Design review of the part built by this model. Coordinates are the model's own, in mm. A direction names the side the tool comes from. Coordinates: 2 decimals unless noted, no trailing zeros. Loops run counter-clockwise (first coordinate to the right, second up) from the corner with the lowest first, then second, coordinate; pieces in that order, holes last.
Q1. Add section A-A on x = -4. Give the boundary of the cut face in (y, z).
Q2. For P1, Ø0.8, axis at x = 57.5, y = -25.5, coming from the -Z side, flat-tipped, find the tip position at first contact; note if it passes through.
Q3. Wall thickness on probe 1 along X at (y, z) = (28, 16.25); probe 2 along Y at (x, z) = (-52, 13.5); probe 3 along Z at (x, y) = (27, -41.5): over which ranges is each line inside the solid? List them lowest first.
Q4. Add section B-B on z = 20.25. Give the boundary of the cut face in (x, y).
Q5. Add section D-D on y = -36. Give the boundary of the cut face in (x, z), and give its area (3 significant figures).
Q6. Draft analysis for pull direction Y (two halves, no side actions). For faces 4 (the face through (-57, -42.7, 15)), 5 (the face through (-57, -8, 17.8)), 6 (the face through (-54, 32, 12.8)), 7 (the face through (0, -50.5, 19)), state which applies: released by +Y, released by -Y, zero draft, split by the parting line, or undercut.
Q7. Machinability: for faces 1 (the face through (1, 34.5, 19)), 2 (the face through (0, -47.7, 19)), 3 (the face through (-57, 26.7, 15)), which of the approach directions +Z, -Z, +X, -X, +Y, -Y give a long, thin tool a straight path to every point of the face, cutting with its end or side? Answer none if there is none.
Q8. Add section C-C on y = -16. Give the boundary of the cut face in (x, z).
```python
from build123d import *

# Parameters (mm, degrees)
SKETCH022_W     = 117
SKETCH022_H     = 85
PAD013_DEPTH    = 5.8
SKETCH023_W     = 95.2
SKETCH023_H     = 58.2
POCKET001_DEPTH = 5.801
SKETCH024_W     = 111.4
SKETCH024_H     = 79.4
POCKET002_DEPTH = 3.8
POCKET008_DEPTH = 5.801
PAD017_DEPTH    = 5
SKETCH044_W     = 2.8
SKETCH044_H     = 3.2
PAD018_DEPTH    = 1.4
SKETCH045_W     = 2.8
SKETCH045_H     = 3.2
PAD019_DEPTH    = 1.4
POCKET016_DEPTH = 85.001
CHAMFER001_SIZE = 1.4


with BuildPart() as part:
    # Sketch022 → Pad013 (new body)
    with BuildSketch(Plane.XY.offset(23.6)):
        with Locations((0.5, -8)):
            Rectangle(SKETCH022_W, SKETCH022_H)
    extrude(amount=-PAD013_DEPTH)

    # Sketch023 (on Face5 of Pad013) → Pocket001 (cut, through all)
    with BuildSketch(Plane.XY.offset(23.6)):
        with Locations((0.9, 0)):
            Rectangle(SKETCH023_W, SKETCH023_H)
    extrude(amount=-POCKET001_DEPTH, mode=Mode.SUBTRACT)

    # Sketch024 (on Face5 of Pocket001) → Pocket002 (cut)
    with BuildSketch(Plane(origin=(0, 0, 17.8), x_dir=(1, 0, 0), z_dir=(0, 0, -1))):
        with Locations((0.5, 8)):
            Rectangle(SKETCH024_W, SKETCH024_H)
    extrude(amount=-POCKET002_DEPTH, mode=Mode.SUBTRACT)

    # Sketch031 (on Face4 of Pocket002) → Pocket008 (cut, through all)
    with BuildSketch(Plane.XY.offset(23.6)):
        with BuildLine():
            Line((-51.4, -33.8), (-41.6, -33.8))
            ThreePointArc((-40.6, -34.8), (-40.892893, -34.092893), (-41.6, -33.8))
            Line((-40.6, -34.8), (-40.6, -44.6))
            ThreePointArc((-41.6, -45.6), (-40.892893, -45.307107), (-40.6, -44.6))
            Line((-41.6, -45.6), (-51.4, -45.6))
            ThreePointArc((-52.4, -44.6), (-52.107107, -45.307107), (-51.4, -45.6))
            Line((-52.4, -44.6), (-52.4, -34.8))
            ThreePointArc((-51.4, -33.8), (-52.107107, -34.092893), (-52.4, -34.8))
        make_face()
        with BuildLine():
            Line((-37.6, -33.8), (-27.8, -33.8))
            ThreePointArc((-26.8, -34.8), (-27.092893, -34.092893), (-27.8, -33.8))
            Line((-26.8, -34.8), (-26.8, -44.6))
            ThreePointArc((-27.8, -45.6), (-27.092893, -45.307107), (-26.8, -44.6))
            Line((-27.8, -45.6), (-37.6, -45.6))
            ThreePointArc((-38.6, -44.6), (-38.307107, -45.307107), (-37.6, -45.6))
            Line((-38.6, -44.6), (-38.6, -34.8))
            ThreePointArc((-37.6, -33.8), (-38.307107, -34.092893), (-38.6, -34.8))
        make_face()
        with BuildLine():
            Line((-9.5, -33.8), (0.3, -33.8))
            ThreePointArc((1.3, -34.8), (1.007107, -34.092893), (0.3, -33.8))
            Line((1.3, -34.8), (1.3, -44.6))
            ThreePointArc((0.3, -45.6), (1.007107, -45.307107), (1.3, -44.6))
            Line((0.3, -45.6), (-9.5, -45.6))
            ThreePointArc((-10.5, -44.6), (-10.207107, -45.307107), (-9.5, -45.6))
            Line((-10.5, -44.6), (-10.5, -34.8))
            ThreePointArc((-9.5, -33.8), (-10.207107, -34.092893), (-10.5, -34.8))
        make_face()
    extrude(amount=-POCKET008_DEPTH, mode=Mode.SUBTRACT)

    # Sketch038 (on Face5 of Pocket008) → Pad017 (join)
    with BuildSketch(Plane(origin=(0, 0, 17.8), x_dir=(1, 0, 0), z_dir=(0, 0, -1))):
        Polygon((-58, 50.5), (-48.2, 50.5), (-48.2, 47.7), (-55.2, 47.7), (-55.2, 42.7), (-58, 42.7), align=None)
        Polygon((59, 50.5), (49.2, 50.5), (49.2, 47.7), (56.2, 47.7), (56.2, 42.7), (59, 42.7), align=None)
        Polygon((59, -34.5), (49.2, -34.5), (49.2, -31.7), (56.2, -31.7), (56.2, -26.7), (59, -26.7), align=None)
        Polygon((-58, -34.5), (-48.2, -34.5), (-48.2, -31.7), (-55.2, -31.7), (-55.2, -26.7), (-58, -26.7), align=None)
    extrude(amount=PAD017_DEPTH)

    # Sketch044 (on Face66 of Pad017) → Pad018 (join)
    with BuildSketch(Plane.YZ.offset(-48.2)):
        with Locations((-49.1, 14.4)):
            Rectangle(SKETCH044_W, SKETCH044_H)
        with Locations((33.1, 14.4)):
            Rectangle(SKETCH044_W, SKETCH044_H)
    extrude(amount=PAD018_DEPTH)

    # Sketch045 (on Face68 of Pad018) → Pad019 (join)
    with BuildSketch(Plane(origin=(49.2, 0, 0), x_dir=(0, -1, 0), z_dir=(-1, 0, 0))):
        with Locations((-33.1, 14.4)):
            Rectangle(SKETCH045_W, SKETCH045_H)
        with Locations((49.1, 14.4)):
            Rectangle(SKETCH045_W, SKETCH045_H)
    extrude(amount=PAD019_DEPTH)

    # Sketch046 (on Face76 of Pad019) → Pocket016 (cut, through all)
    with BuildSketch(Plane.XZ.offset(50.5)):
        Polygon((-48.2, 16), (-46.8, 16), (-46.8, 14.4), align=None)
        Polygon((47.8, 16), (49.2, 16), (47.8, 14.4), align=None)
    extrude(amount=-POCKET016_DEPTH, mode=Mode.SUBTRACT)

    # Chamfer001
    chamfer001_edges = [part.edges().sort_by_distance(p)[0] for p in [
        (0.9, 29.1, 23.6),
        (-46.7, 0, 23.6),
        (48.5, 0, 23.6),
        (0.9, -29.1, 23.6),
    ]]
    chamfer(chamfer001_edges, length=CHAMFER001_SIZE)


solid = part.part
```
Entries:
1. outline: (-50.5, 17.8) - (-47.7, 17.8) - (-47.7, 21.6) - (-45.6, 21.6) - (-45.6, 23.6) - (-50.5, 23.6) - close; (-33.8, 21.6) - (-29.1, 21.6) - (-29.1, 22.2) - (-30.5, 23.6) - (-33.8, 23.6) - close; (29.1, 21.6) - (31.7, 21.6) - (31.7, 17.8) - (34.5, 17.8) - (34.5, 23.6) - (30.5, 23.6) - (29.1, 22.2) - close
2. P1: stops at z = 17.8
3. probe 1: x = -58 to -55.2, 56.2 to 59
3. probe 2: y = -50.5 to -47.7, 31.7 to 34.5
3. probe 3: z = 21.6 to 23.6
4. outline: (-58, -50.5) - (59, -50.5) - (59, 34.5) - (-58, 34.5) - close; hole (-55.2, -47.7) - (56.2, -47.7) - (56.2, 31.7) - (-55.2, 31.7) - close
5. outline: (-58, 17.8) - (-55.2, 17.8) - (-55.2, 21.6) - (-52.4, 21.6) - (-52.4, 23.6) - (-58, 23.6) - close; (-40.6, 21.6) - (-38.6, 21.6) - (-38.6, 23.6) - (-40.6, 23.6) - close; (-26.8, 21.6) - (-10.5, 21.6) - (-10.5, 23.6) - (-26.8, 23.6) - close; (1.3, 21.6) - (56.2, 21.6) - (56.2, 17.8) - (59, 17.8) - (59, 23.6) - (1.3, 23.6) - close
5. area: 184 mm2
6. face 4: undercut
6. face 5: undercut
6. face 6: zero draft
6. face 7: released by -Y
7. face 1: +Z, -Z, +X, -X, +Y
7. face 2: -Z
7. face 3: -Z, +X, -X
8. outline: (-58, 17.8) - (-55.2, 17.8) - (-55.2, 21.6) - (-46.7, 21.6) - (-46.7, 22.2) - (-48.1, 23.6) - (-58, 23.6) - close; (48.5, 21.6) - (56.2, 21.6) - (56.2, 17.8) - (59, 17.8) - (59, 23.6) - (49.9, 23.6) - (48.5, 22.2) - close
